```python
from build123d import *

# Parameters (mm, degrees)
SKETCH1_R            = 8.525
BOSS_EXTRUDE11_DEPTH = 4
SKETCH20_R           = 8.525
BOSS_EXTRUDE12_DEPTH = 4
SKETCH21_R           = 9.5
BOSS_EXTRUDE13_DEPTH = 1.5
SKETCH22_R           = 8.525
BOSS_EXTRUDE14_DEPTH = 5.6
BOSS_EXTRUDE15_START = 14.75
SKETCH30_R           = 8.525
BOSS_EXTRUDE15_DEPTH = 14.75
SKETCH33_R           = 2.1
CUT_EXTRUDE14_DEPTH  = 5.8
BOSS_EXTRUDE16_START = 1.25
SKETCH35_R           = 9.5
BOSS_EXTRUDE16_DEPTH = 1.25
SKETCH36_R           = 1.6
CUT_EXTRUDE15_DEPTH  = 29.85
CIRPATTERN1_COUNT    = 2
SKETCH43_R           = 1.55
CUT_EXTRUDE20_DEPTH  = 29.85
SKETCH44_R           = 2
CUT_EXTRUDE21_DEPTH  = 4
CUT_EXTRUDE22_DEPTH  = 1.7
CUT_EXTRUDE23_DEPTH  = 3
SKETCH47_W           = 28.870202412
SKETCH47_H           = 25.831233738
CUT_EXTRUDE24_DEPTH  = 18.75
SKETCH48_W           = 6
SKETCH48_H           = 6
BOSS_EXTRUDE17_DEPTH = 3
FILLET1_R            = 0.6
CHAMFER1_SIZE        = 1.7


with BuildPart() as part:
    # Sketch1 → Boss-Extrude11 (new body)
    with BuildSketch(Plane(origin=(0, 0, 0), x_dir=(1, 0, 0), z_dir=(0, 1, 0))):
        with Locations(Location((0, 0, 0), (0, 0, 270))):
            Circle(SKETCH1_R)
    extrude(amount=BOSS_EXTRUDE11_DEPTH)

    # Sketch20 → Boss-Extrude12 (add)
    with BuildSketch(Plane(origin=(0, 4, 0), x_dir=(1, 0, 0), z_dir=(0, 1, 0))):
        with Locations(Location((1.2, 0, 0), (0, 0, 94.035884191))):
            Circle(SKETCH20_R)
    extrude(amount=BOSS_EXTRUDE12_DEPTH)

    # Sketch21 → Boss-Extrude13 (add)
    with BuildSketch(Plane(origin=(0, 8, 0), x_dir=(1, 0, 0), z_dir=(0, 1, 0))):
        with Locations(Location((0.6, 0, 0), (0, 0, 270))):
            Circle(SKETCH21_R)
    extrude(amount=BOSS_EXTRUDE13_DEPTH)

    # Sketch22 → Boss-Extrude14 (add)
    with BuildSketch(Plane(origin=(0, 9.5, 0), x_dir=(1, 0, 0), z_dir=(0, 1, 0))):
        with Locations(Location((0.6, 0, 0), (0, 0, 270))):
            Circle(SKETCH22_R)
    extrude(amount=BOSS_EXTRUDE14_DEPTH)

    # Sketch30 → Boss-Extrude15 (add)
    with BuildSketch(Plane.XZ.offset(BOSS_EXTRUDE15_START)):
        with Locations(Location((0.6, 0, 0), (0, 0, 90))):
            Circle(SKETCH30_R)
    extrude(amount=-BOSS_EXTRUDE15_DEPTH)

    # Sketch33 → Cut-Extrude14 (cut)
    with BuildSketch(Plane.XZ.offset(14.75)):
        with Locations(Location((0.6, 0, 0), (0, 0, 270))):
            Circle(SKETCH33_R)
    extrude(amount=-CUT_EXTRUDE14_DEPTH, mode=Mode.SUBTRACT)

    # Sketch35 → Boss-Extrude16 (add)
    with BuildSketch(Plane.XZ.offset(BOSS_EXTRUDE16_START)):
        with Locations(Location((0.6, 0, 0), (0, 0, 90))):
            Circle(SKETCH35_R)
    extrude(amount=-BOSS_EXTRUDE16_DEPTH)

    # Sketch36 → Cut-Extrude15 (cut)
    with BuildSketch(Plane.XZ.offset(14.75)):
        with Locations(Location((0.6, 6, 0), (0, 0, 270))):
            Circle(SKETCH36_R)
    cut_extrude15 = extrude(amount=-CUT_EXTRUDE15_DEPTH, mode=Mode.SUBTRACT)

    # CirPattern1: Cut-Extrude15 ×2 about axis
    cirpattern1_axis = Axis((0.6, 0, 0), (0, 1, 0))
    for i in range(1, CIRPATTERN1_COUNT):
        add(cut_extrude15.rotate(cirpattern1_axis, i * 360 / CIRPATTERN1_COUNT), mode=Mode.SUBTRACT)

    # Sketch43 → Cut-Extrude20 (cut)
    with BuildSketch(Plane.XZ.offset(14.75)):
        with Locations(Location((-4.9, 0, 0), (0, 0, 270))):
            Circle(SKETCH43_R)
        with Locations(Location((6.1, 0, 0), (0, 0, 270))):
            Circle(SKETCH43_R)
    extrude(amount=-CUT_EXTRUDE20_DEPTH, mode=Mode.SUBTRACT)

    # Sketch44 → Cut-Extrude21 (cut)
    with BuildSketch(Plane(origin=(0, 15.1, 0), x_dir=(1, 0, 0), z_dir=(0, 1, 0))):
        with Locations(Location((-4.9, 0, 0), (0, 0, 270))):
            Circle(SKETCH44_R)
        with Locations(Location((6.1, 0, 0), (0, 0, 270))):
            Circle(SKETCH44_R)
    extrude(amount=-CUT_EXTRUDE21_DEPTH, mode=Mode.SUBTRACT)

    # Sketch45 → Cut-Extrude22 (cut)
    with BuildSketch(Plane(origin=(0, 15.1, 0), x_dir=(1, 0, 0), z_dir=(0, 1, 0))):
        with BuildLine():
            Line((-2.9, -6), (-2.9, -10.872564071))
            Line((-2.9, -10.872564071), (4.1, -10.872564071))
            Line((4.1, -10.872564071), (4.1, -6))
            ThreePointArc((4.1, -6), (0.6, -2.5), (-2.9, -6))
        make_face()
        with BuildLine():
            Line((-2.9, 6), (-2.9, 11.42214608))
            Line((-2.9, 11.42214608), (4.1, 11.42214608))
            Line((4.1, 11.42214608), (4.1, 6))
            ThreePointArc((4.1, 6), (0.6, 2.5), (-2.9, 6))
        make_face()
    extrude(amount=-CUT_EXTRUDE22_DEPTH, mode=Mode.SUBTRACT)

    # Sketch46 → Cut-Extrude23 (cut)
    with BuildSketch(Plane.XZ.offset(14.75)):
        with BuildLine():
            Line((-4.9, 3), (-9.719928829, 3))
            Line((-9.719928829, 3), (-9.719928829, -3))
            Line((-9.719928829, -3), (-4.9, -3))
            ThreePointArc((-4.9, -3), (-1.9, 0), (-4.9, 3))
        make_face()
        with BuildLine():
            Line((6.1, 3), (10.889396495, 3))
            Line((10.889396495, 3), (10.889396495, -3))
            Line((10.889396495, -3), (6.1, -3))
            ThreePointArc((6.1, -3), (3.1, 0), (6.1, 3))
        make_face()
    extrude(amount=-CUT_EXTRUDE23_DEPTH, mode=Mode.SUBTRACT)

    # Sketch47 → Cut-Extrude24 (cut)
    with BuildSketch(Plane.XZ.offset(14.75)):
        with Locations((1.011527008, 0.205763504)):
            Rectangle(SKETCH47_W, SKETCH47_H)
    extrude(amount=-CUT_EXTRUDE24_DEPTH, mode=Mode.SUBTRACT)

    # Sketch48 → Boss-Extrude17 (add)
    with BuildSketch(Plane.XZ.offset(-4)):
        with Locations((1.2, 0)):
            Rectangle(SKETCH48_W, SKETCH48_H)
    extrude(amount=BOSS_EXTRUDE17_DEPTH)

    # Fillet1
    fillet1_edges = [part.edges().sort_by_distance(p)[0] for p in [
        (-1.8, 1, 0),
        (1.2, 1, -3),
        (4.2, 1, 0),
        (1.2, 1, 3),
    ]]
    fillet(fillet1_edges, radius=FILLET1_R)

    # Chamfer1
    chamfer1_edges = [part.edges().sort_by_distance(p)[0] for p in [
        (4.1, 13.4, 6.886696058),
        (-2.9, 13.4, 6.886696058),
        (-2.9, 13.4, -6.886696058),
        (4.1, 13.4, -6.886696058),
        (0.6, 13.4, 2.5),
        (0.6, 13.4, -2.5),
    ]]
    chamfer(chamfer1_edges, length=CHAMFER1_SIZE - 0.0001)  # a hair under: the kernel refuses the full size


solid = part.part
```
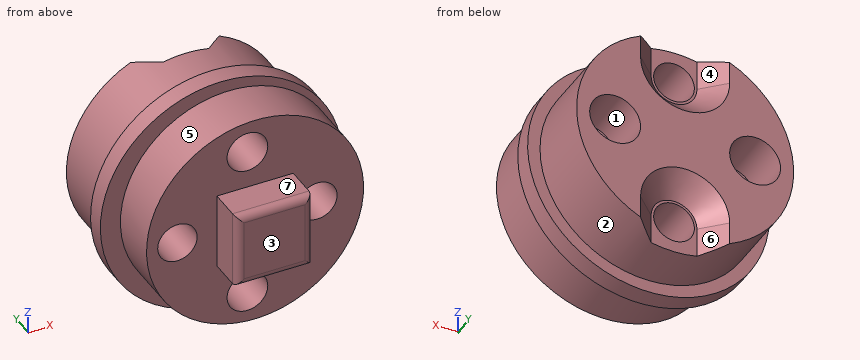
Input: part model. Units: mm. Frame: model coordinates. Face numbers are marked on the shaded views. A direction names the side the tool comes from. Give positions to 0.01 mm unless a question says otherwise; leave off trailing zeros. Write each loop counter-clockwise with the first axis right and the second up, starting at its lowest first coordinate (ties: lowest second). Pieces come first, ordered by that corner, then holes. Notation, with made-up numbers: (-4, 78) - (47, 78) arc R31 cw to (47, 110) - close; hole circle Ø3 at (87.25, 36). An arc over 180 degrees is marked (long way). Write item = value, one per line. Start each with the question number.
1) Material intervals for L1, parallel to X at y = 12.25, z = 0 (3 decimals); L2, parallel to Z at x = 0.5, y = 10.75; L3, parallel to X at y = 8.25, z = 0, sorted ascending. Write a range as [from, to].
2) Cut plane C-C (y = 10). Return loops of the section in (x, z) (3 decimals).
3) Cut plane D-D (y = 14). Return loops of the section in (x, z) (3 decimals), and give its area (3 significant figures).
4) Reachability of the marked faces 4, 5, 6 and 7 from +Z, -Z, +X, -X, +Y, -Y: full face, straight path, thin tool, end or side. Return the list, or none.
5) Cut plane A-A (x = 6.1). Return loops of the section in (y, z).
6) Cut plane B-B (z = 0.5). Give the number of separate pieces and of enclosed holes in the cut face, and give its area (3 significant figures).
7) Draft query along X for the marked faces 1, 2 and 3. Return one class per face: pulls with the +X half, pulls with the -X half, needs draft (parallel to the pull), parting line crosses it, or undercut.
8) Pin query (flat end, axial travel): pin 1 (1.2 mm diameter, centred on x = 6.5, z = 1, fed in from +Y); pin 2 (5 mm diameter, centred on x = -4.9, z = 0, fed in from -Y); pin 3 (1.5 mm diameter, centred on x = -5, z = 7, fed in from +Y); pin 4 (4 mm diameter, centred on x = 0.5, z = -5.5, fed in from +Y). Return the tip coordinate at first contact, or that it passes through.
Answers follow:
q1.L1 = [-7.925, -6.9], [-2.9, 4.1], [8.1, 9.125]
q1.L2 = [-8.52, -7.6], [-4.4, 4.4], [7.6, 8.52]
q1.L3 = [-8.9, -6.45], [-3.35, 4.55], [7.65, 10.1]
q2.outline = circle Ø17.05 at (0.6, 0); hole circle Ø3.1 at (-4.9, 0); hole circle Ø3.2 at (0.6, -6); hole circle Ø3.2 at (0.6, 6); hole circle Ø3.1 at (6.1, 0)
q3.outline = (-1.8, -8.18) - (-1.8, -6) arc R2.4 cw to (3, -6) - (3, -8.18) arc R8.525 ccw to (3, 8.18) - (3, 6) arc R2.4 cw to (-1.8, 6) - (-1.8, 8.18) arc R8.525 ccw to start; hole circle Ø4 at (-4.9, 0); hole circle Ø4 at (6.1, 0)
q3.area = 162 mm^2
q4.face_4 = +Z, +Y
q4.face_5 = -Y
q4.face_6 = -Z, +Y
q4.face_7 = +Z, +X, -X, -Y
q5.outline = (4, -6.98) - (8, -6.98) - (8, -7.75) - (9.5, -7.75) - (9.5, -6.51) - (15.1, -6.51) - (15.1, -2) - (11.1, -2) - (11.1, -1.55) - (4, -1.55) - close; (4, 1.55) - (11.1, 1.55) - (11.1, 2) - (15.1, 2) - (15.1, 6.51) - (9.5, 6.51) - (9.5, 7.75) - (8, 7.75) - (8, 6.98) - (4, 6.98) - close
q6.separate_pieces = 3
q6.enclosed_holes = 0
q6.area = 137 mm^2
q7.face_1 = undercut
q7.face_2 = parting line crosses it
q7.face_3 = needs draft
q8.pin_1 = 11.1
q8.pin_2 = 4
q8.pin_3 = 15.1
q8.pin_4 = 14.11
